Read the model definition and answer for the solid it produces. Units are mm, in the model's axes. A direction names the side the tool comes from. Give positions to 0.01 mm unless a question says otherwise; leave off trailing zeros. Order: outer loops, then holes, each group sorted by start corner. A loop starts at its lowest first (then second) coordinate and runs counter-clockwise, first axis right, second up. Notation, with made-up numbers: (-33.5, -29) - (2.5, -29) arc R27 cw to (2.5, 6) - close; hole circle Ø10 at (72.5, -33). An arc over 180 degrees is marked (long way). Write each question's results on one line, items separated by ' | '.
from build123d import *

# Parameters (mm, degrees)
SKETCH1_R                                      = 49.53
BOSS_EXTRUDE1_DEPTH                            = 3.175
SKETCH2_R                                      = 47.625
BOSS_EXTRUDE2_DEPTH                            = 3.175
SKETCH3_R                                      = 3.175
CUT_EXTRUDE1_DEPTH                             = 71.33323752
SKETCH5_R                                      = 3.175
CUT_EXTRUDE2_DEPTH                             = 71.33323752
CSK_FOR_8_FLAT_HEAD_MACHINE_SCREW2_D           = 4.4958
CSK_FOR_8_FLAT_HEAD_MACHINE_SCREW2_CSINK_D     = 8.4328
CSK_FOR_8_FLAT_HEAD_MACHINE_SCREW2_CSINK_ANGLE = 82
CIRPATTERN1_COUNT                              = 4
F_8_CLEARANCE_HOLE1_D                          = 4.4958
F_4_CLEARANCE_HOLE1_D                          = 3.2639


with BuildPart() as part:
    # Sketch1 → Boss-Extrude1 (new body)
    with BuildSketch(Plane(origin=(0, 0, 0), x_dir=(1, 0, 0), z_dir=(0, 1, 0))):
        with Locations(Location((0, 0, 0), (0, 0, 270))):
            Circle(SKETCH1_R)
    extrude(amount=BOSS_EXTRUDE1_DEPTH)

    # Sketch2 → Boss-Extrude2 (add)
    with BuildSketch(Plane(origin=(0, 3.175, 0), x_dir=(1, 0, 0), z_dir=(0, 1, 0))):
        with Locations(Location((0, 0, 0), (0, 0, 270))):
            Circle(SKETCH2_R)
    extrude(amount=BOSS_EXTRUDE2_DEPTH)

    # Sketch3 → Cut-Extrude1 (cut, through all)
    with BuildSketch(Plane(origin=(0, 6.35, 0), x_dir=(1, 0, 0), z_dir=(0, 1, 0))):
        with Locations(Location((-38.1, 0, 0), (0, 0, 270))):
            Circle(SKETCH3_R)
        with Locations(Location((38.1, 0, 0), (0, 0, 270))):
            Circle(SKETCH3_R)
    extrude(amount=-CUT_EXTRUDE1_DEPTH, mode=Mode.SUBTRACT)

    # Sketch5 → Cut-Extrude2 (cut, through all)
    with BuildSketch(Plane(origin=(0, 6.35, 0), x_dir=(1, 0, 0), z_dir=(0, 1, 0))):
        with Locations(Location((0, 0, 0), (0, 0, 270))):
            Circle(SKETCH5_R)
    extrude(amount=-CUT_EXTRUDE2_DEPTH, mode=Mode.SUBTRACT)

    # CSK for #8 Flat Head Machine Screw2 (through all)
    with Locations(Plane(origin=(0, 0, 0), x_dir=(-1, 0, 0), z_dir=(0, -1, 0))):
        with Locations((31.169774814, -30.940594366)):
            csk_for_8_flat_head_machine_screw2 = CounterSinkHole(CSK_FOR_8_FLAT_HEAD_MACHINE_SCREW2_D / 2, CSK_FOR_8_FLAT_HEAD_MACHINE_SCREW2_CSINK_D / 2, counter_sink_angle=CSK_FOR_8_FLAT_HEAD_MACHINE_SCREW2_CSINK_ANGLE)

    # CirPattern1: CSK for #8 Flat Head Machine Screw2 ×4 about axis
    cirpattern1_axis = Axis((0, 0, 0), (0, 1, 0))
    for i in range(1, CIRPATTERN1_COUNT):
        add(csk_for_8_flat_head_machine_screw2.rotate(cirpattern1_axis, i * 360 / CIRPATTERN1_COUNT), mode=Mode.SUBTRACT)

    # #8 Clearance Hole1 (through all)
    with Locations(Plane(origin=(0, 0, 0), x_dir=(-1, 0, 0), z_dir=(0, -1, 0))):
        with Locations((11.293505133, 31.028650338), (-11.293505133, -31.028650338)):
            Hole(F_8_CLEARANCE_HOLE1_D / 2)

    # #4 Clearance Hole1 (through all)
    with Locations(Plane(origin=(0, 0, 0), x_dir=(-1, 0, 0), z_dir=(0, -1, 0))):
        with Locations((-15.929774814, 19.783889264), (15.929774814, -19.783889264), (-15.929774814, 29.943889264), (15.929774814, -29.943889264)):
            Hole(F_4_CLEARANCE_HOLE1_D / 2)


solid = part.part
(1) Each of these flat-tipped pins is pushed along its axis until it touches: pin 1 (1 mm diameter, centred on x = 38, y = 3.5, fed in from -Z); pin 2 (3 mm diameter, centred on x = 5.5, y = 1.5, fed in from -Z); pin 3 (5 mm diameter, centred on x = -31.17, z = 30.94, fed in from -Y). Where does it stop, or does it pass through?
Conclusion:
pin 1: z = -32.22 | pin 2: z = -49.37 | pin 3: y = 1.97
(2) For faces 4 (the face through (-46.492, 4.74, -10.324)), 5 (the face through (17.437, 3.219, -19.159)), determine the directions among +Z, -Z, +X, -X, +Y, -Y from which every point of the face is accessible in a straight line to the end or side of a thin tool.
Conclusion:
face 4: +Y | face 5: +Y, -Y
(3) Section D-D (y = 5) is taken. State how many separate pieces and enclosed holes the cut face has, plus the area to 3 significant figures.
Conclusion:
separate pieces: 1 | enclosed holes: 13 | area: 6,900 mm^2
(4) The mould has two halves that part along Z. Classify faces 1 (the face through (-10, 0, -1)), 2 (the face through (14.88, 1.57, 47.24)), 3 (the face through (35, 3.22, -0.69)): pulls with the +Z half, pulls with the -Z half, needs draft (parallel to the pull), parting line crosses it, or undercut.
Conclusion:
face 1: needs draft | face 2: parting line crosses it | face 3: undercut
(5) Section B-B (x = 0) is taken. Give the vertices of the cut face in (y, z) (3 decimals).
Conclusion:
outline: (0, -49.53) - (3.175, -49.53) - (3.175, -47.625) - (6.35, -47.625) - (6.35, -3.175) - (0, -3.175) - close; (0, 3.175) - (6.35, 3.175) - (6.35, 47.625) - (3.175, 47.625) - (3.175, 49.53) - (0, 49.53) - close
(6) Section A-A (z = 0) is taken. Give the vertices of the cut face in (x, y) (3 decimals).
Conclusion:
outline: (-49.53, 0) - (-41.275, 0) - (-41.275, 6.35) - (-47.625, 6.35) - (-47.625, 3.175) - (-49.53, 3.175) - close; (-34.925, 0) - (-3.175, 0) - (-3.175, 6.35) - (-34.925, 6.35) - close; (3.175, 0) - (34.925, 0) - (34.925, 6.35) - (3.175, 6.35) - close; (41.275, 0) - (49.53, 0) - (49.53, 3.175) - (47.625, 3.175) - (47.625, 6.35) - (41.275, 6.35) - close
(7) Consider probe 1 along X at (y, z) = (1.25, 29.5); probe 2 along X at (y, z) = (5.25, -20.5); probe 3 along Y at (x, z) = (-44.5, 18.5) (3 decimals). Determine where each line is inside the solid, lowest interval first. Write a range as [from, to].
Conclusion:
probe 1: [-39.79, -33.95], [-28.39, -17.5], [-14.36, 9.65], [12.94, 28.29], [33.59, 39.79] | probe 2: [-42.99, 14.46], [17.4, 42.99] | probe 3: [0, 3.175]
(8) Section C-C (x = 15.5) is taken. Give the vertices of the cut face in (y, z) (3 decimals).
Conclusion:
outline: (0, -47.042) - (3.175, -47.042) - (3.175, -45.032) - (6.35, -45.032) - (6.35, -31.518) - (0, -31.518) - close; (0, -28.37) - (6.35, -28.37) - (6.35, -21.358) - (0, -21.358) - close; (0, -18.21) - (6.35, -18.21) - (6.35, 45.032) - (3.175, 45.032) - (3.175, 47.042) - (0, 47.042) - close
